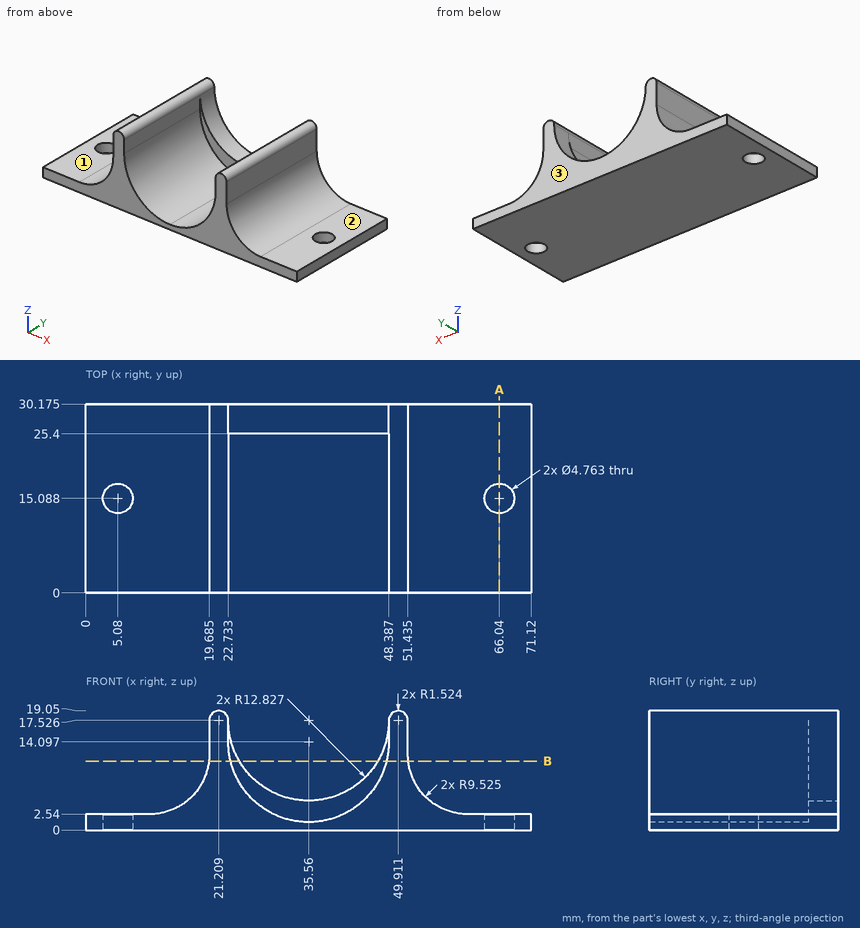
Here's the drawing with two shaded views (mm, measured from the low corner). I have some questions. A direction names the side the tool comes from. Give positions to 0.01 mm unless a question says otherwise; leave off trailing zeros. Loops run counter-clockwise (first coordinate to the right, second up) from the corner with the lowest first, then second, coordinate; pieces in that order, holes last. Notation, with made-up numbers: (65.25, 37.25) - (89.25, 37.25) arc R15 cw to (89.25, 54.25) - close; hole circle Ø11 at (25.5, 67.25). An arc over 180 degrees is marked (long way). Answer in a Markdown table with one row per item. Add a question column.
Q1. For pin 1 (1.6 mm diameter, centred on y = 10.5, z = 15, fed in from +X) (1 decimal); pin 2 (3 mm diameter, centred on y = 23.5, z = 11.5, fed in from +X); pin 3 (3 mm diameter, centred on x = 64.5, y = 14, fed in from +Z), each with a flat end and sliding along its axis, tell me the tip position at first contact or that it passes through.
Q2. Please list where these lines run through material, in increasing order: L1, parallel to X at y = 21, z = 16.75 (1 decimal); L2, parallel to Y at x = 5.08, z = 1.35 (1 decimal); L3, parallel to Z at x = 7.5, y = 24.5. Write a range as from..to.
Q3. Which directions (+Z, -Z, +X, -X, +Y, -Y) give clear straight access to the entire face, cutting with the end or side of a thin tool? Please do the marked faces 1, 2 and 3.
Q4. If we section it at A-A (x = 66.04): List the corners of the cut face in (y, z) for me (1 decimal).
Q5. If we section it at B-B (z = 11): List the corners of the cut face in (x, y) for me (1 decimal), plus the area to 3 significant figures.
The answers:
| question | item | result |
|---|---|---|
| 1 | pin 1 | stops at x = 51.4 |
| 1 | pin 2 | stops at x = 51.66 |
| 1 | pin 3 | stops at z = 2.54 |
| 2 | L1 | x = 19.7..22.7, 48.4..51.4 |
| 2 | L2 | y = 0..12.7, 17.5..30.2 |
| 2 | L3 | z = 0..2.54 |
| 3 | face 1 | +Z, -X, +Y, -Y |
| 3 | face 2 | +Z, +X, +Y, -Y |
| 3 | face 3 | +Z, -Z, +X, -X, +Y |
| 4 | outline | (0, 0) - (12.7, 0) - (12.7, 2.5) - (0, 2.5) - close; (17.5, 0) - (30.2, 0) - (30.2, 2.5) - (17.5, 2.5) - close |
| 5 | outline | (19.6, 0) - (23.1, 0) - (23.1, 25.4) - (24.5, 25.4) - (24.5, 30.2) - (19.6, 30.2) - close; (46.6, 25.4) - (48, 25.4) - (48, 0) - (51.5, 0) - (51.5, 30.2) - (46.6, 30.2) - close |
| 5 | area | 224 mm^2 |
